from build123d import *

# Parameters (mm, degrees)
SKETCH1_R           = 63.5
SKETCH1_R_2         = 20
BOSS_EXTRUDE1_DEPTH = 50.8
SKETCH3_R           = 76.2
SKETCH3_R_2         = 5.1
SKETCH3_R_3         = 1.5
BOSS_EXTRUDE2_DEPTH = 5
SKETCH4_R           = 76.2
SKETCH4_R_2         = 20
BOSS_EXTRUDE3_DEPTH = 5
SKETCH5_R           = 11.1
CUT_EXTRUDE1_DEPTH  = 1.2
SKETCH6_R           = 1.5875
BOSS_EXTRUDE4_DEPTH = 2.5


with BuildPart() as part:
    # Sketch1 → Boss-Extrude1 (new body)
    with BuildSketch(Plane.XY):
        Circle(SKETCH1_R)
        Circle(SKETCH1_R_2, mode=Mode.SUBTRACT)
    extrude(amount=BOSS_EXTRUDE1_DEPTH)

    # Sketch3 → Boss-Extrude2 (add)
    with BuildSketch(Plane.XY):
        Circle(SKETCH3_R)
        Circle(SKETCH3_R_2, mode=Mode.SUBTRACT)
        with Locations((0, 8)):
            Circle(SKETCH3_R_3, mode=Mode.SUBTRACT)
        with Locations((8, 0)):
            Circle(SKETCH3_R_3, mode=Mode.SUBTRACT)
        with Locations((0, -8)):
            Circle(SKETCH3_R_3, mode=Mode.SUBTRACT)
        with Locations((-8, 0)):
            Circle(SKETCH3_R_3, mode=Mode.SUBTRACT)
    extrude(amount=BOSS_EXTRUDE2_DEPTH)

    # Sketch4 → Boss-Extrude3 (add)
    with BuildSketch(Plane.XY.offset(50.8)):
        Circle(SKETCH4_R)
        Circle(SKETCH4_R_2, mode=Mode.SUBTRACT)
    extrude(amount=BOSS_EXTRUDE3_DEPTH)

    # Sketch5 → Cut-Extrude1 (cut)
    with BuildSketch(Plane(origin=(0, 0, 0), x_dir=(-1, 0, 0), z_dir=(0, 0, -1))):
        Circle(SKETCH5_R)
    extrude(amount=-CUT_EXTRUDE1_DEPTH, mode=Mode.SUBTRACT)

    # Sketch6 → Boss-Extrude4 (add, symmetric)
    with BuildSketch(Plane(origin=(0, 0, 0), x_dir=(1, 0, 0), z_dir=(0, 1, 0))):
        with BuildLine():
            Line((-59.663256535, -29.884375), (-59.663256535, -24.328125))
            Line((-59.663256535, -24.328125), (-67.336743465, -24.328125))
            ThreePointArc((-67.336743465, -24.328125), (-70.114868465, -27.10625), (-67.336743465, -29.884375))
            Line((-67.336743465, -29.884375), (-59.663256535, -29.884375))
        make_face()
        with Locations(Location((-67.336743465, -27.10625, 0), (0, 0, 270))):
            Circle(SKETCH6_R, mode=Mode.SUBTRACT)
    extrude(amount=BOSS_EXTRUDE4_DEPTH, both=True)


solid = part.part
Read the model definition and answer for the solid it produces. Units are mm, in the model's axes. A direction names the side the tool comes from. Coordinates: 2 decimals unless noted, no trailing zeros. Loops run counter-clockwise (first coordinate to the right, second up) from the corner with the lowest first, then second, coordinate; pieces in that order, holes last. Notation, with made-up numbers: (53, 28.25) -> (65, 28.25) arc R22 ccw to (65, 45.25) -> close; hole circle Ø8 at (3.25, 76.5). An arc over 180 degrees is marked (long way). Write item = value, one per line. Start each with the question number.
1) The part is cut by section A-A, the plane z = 45.5. Determine the outline of the cut face in (x, y), plus the area to 3 significant figures.
2) The part is cut by section B-B, the plane x = -61. Determine the outline of the cut face in (y, z).
3) For faces 1 (the face through (-29, 57, 5)), 2 (the face through (-65, -2.5, 27)), 3 (the face through (-5, -2, 1.2)), 4 (the face through (4, -4, 5)), 5 (the face through (-65, 2.5, 27)), determine the directions among +Z, -Z, +X, -X, +Y, -Y from which every point of the face is accessible in a straight line to the end or side of a thin tool.
4) Find the intervals of material crossed by L1, parallel to Y at x = 0, z = 3.55; L2, parallel to X at y = 0, z = 30; L3, parallel to Y at x = 0, z = 0.7, in increasing order. Write a range as from..to.
5) The part is cut by section C-C, the plane y = -43. Determine the outline of the cut face in (x, z).
6) The mould has two halves that part along Y. Classify faces 6 (the face through (-4.336, -19.524, 30.044)), 7 (the face through (-65, 0, 29.884)), 8 (the face through (-13.77, -61.99, 27.58)): pulls with the +Y half, pulls with the -Y half, needs draft (parallel to the pull), parting line crosses it, or undercut.
7) Given P1, Ø20, axis at x = -7.5, y = 1.5, coming from the +Z side; P2, Ø2.5, axis at x = 8, y = 0, coming from the -Z side; P3, Ø5, axis at x = 0, y = 8, coming from the -Z side; P4, Ø1, axis at y = -17, z = 10.5, coming from the +X side, each flat-ended and moving along its own axis, determine where each tip first touches the part or whether it passes through.
Result:
q1.outline = circle Ø127 at (0, 0); hole circle Ø40 at (0, 0)
q1.area = 11,400 mm²
q2.outline = (-45.67, 0) -> (45.67, 0) -> (45.67, 5) -> (17.64, 5) -> (17.64, 50.8) -> (45.67, 50.8) -> (45.67, 55.8) -> (-45.67, 55.8) -> (-45.67, 50.8) -> (-17.64, 50.8) -> (-17.64, 5) -> (-45.67, 5) -> close
q3.face_1 = none
q3.face_2 = -X, -Y
q3.face_3 = -Z
q3.face_4 = +Z
q3.face_5 = -X, +Y
q4.L1 = -76.2..-9.5, -6.5..-5.1, 5.1..6.5, 9.5..76.2
q4.L2 = -63.5..-20, 20..63.5
q4.L3 = -76.2..-11.1, 11.1..76.2
q5.outline = (-62.91, 0) -> (62.91, 0) -> (62.91, 5) -> (46.73, 5) -> (46.73, 50.8) -> (62.91, 50.8) -> (62.91, 55.8) -> (-62.91, 55.8) -> (-62.91, 50.8) -> (-46.73, 50.8) -> (-46.73, 5) -> (-62.91, 5) -> close
q6.face_6 = undercut
q6.face_7 = needs draft
q6.face_8 = parting line crosses it
q7.P1 = 5
q7.P2 = through
q7.P3 = 1.2
q7.P4 = 61.32
